Autodesk Inventor part; units mm, degrees
ref_plane "YZ Plane" through (0, 0, 0) normal (1, 0, 0) x (0, 1, 0)
ref_plane "XZ Plane" through (0, 0, 0) normal (0, 1, 0) x (-1, 0, 0)
ref_plane "XY Plane" through (0, 0, 0) normal (0, 0, 1) x (1, 0, 0)
sketch "Boceto1" plane through (0, 0, 0) normal (0, 0, 1) x (1, 0, 0)
  line L0 (48.5, -35) -> (48.5, 68)
  line L1 (48.5, 65) -> (35.5, 65)
  line L2 (-48.5, 68) -> (-48.5, -35)
  line L3 (-48.5, -32) -> (48.5, -32)
  line L4 (-48.5, -32) -> (48.5, -32)
  line L5 (48.5, -32) -> (48.5, 65)
  line L6 (48.5, 65) -> (-48.5, 65)
  line L7 (-48.5, 65) -> (-48.5, -32)
  point P0 (0, 0)
  point P1 (-48.5, 65)
extrude "Extrusión1" add sketch "Boceto1" along normal blind 3
sketch "Boceto5" plane through (0, 0, 0) normal (0, 0, -1) x (-1, 0, 0)
  line L0 (11.3801, -12.7901) -> (-11.3717, -12.7901)
  line L1 (19.791, -21.201) -> (5.6217, -7.0317)
  line L2 (-5.6132, -7.0317) -> (-19.7826, -21.201)
  line L3 (9.0613, -10.4713) -> (-9.0529, -10.4713)
  arc A0 (-19.7826, -21.201) -> (19.791, -21.201) centre (0.0042, 0) ccw
  point P0 (0, 0)
extrude "Extrusión5" cut sketch "Boceto5" against normal through all
sketch "Boceto6" plane through (0, 0, 0) normal (0, 0, -1) x (-1, 0, 0)
  arc A0 (-19.7826, -21.201) -> (19.791, -21.201) centre (0.0042, 0) ccw
  circle A1 centre (-38.9983, 5) radius 1.25
  circle A2 centre (-38.9983, 5) radius 1.25
  circle A3 centre (-38.9983, -5) radius 1.25
  circle A4 centre (39.0017, 5) radius 1.25
  circle A5 centre (39.0017, 5) radius 1.25
  circle A6 centre (39.0017, -5) radius 1.25
  point P0 (0, 0)
hole "Agujero1" at (-0.0042, 0, 0) direction (0, 0, 1) diameter 8.1 end through all
sketch "Boceto7" plane through (0, 0, 0) normal (0, 0, -1) x (-1, 0, 0)
  circle A0 centre (25.3722, 27.0019) radius 1.5
  circle A1 centre (0.0042, 0) radius 4.05
  arc A2 (-19.7826, -21.201) -> (19.791, -21.201) centre (0.0042, 0) ccw
  line L0 (-19.7826, -21.201) -> (-9.0529, -10.4713)
  line L1 (-9.0529, -10.4713) -> (9.0613, -10.4713)
  line L2 (9.0613, -10.4713) -> (19.791, -21.201)
  line L3 (48.5, 65) -> (48.5, -32)
  line L4 (-48.5, 65) -> (48.5, 65)
  line L5 (-48.5, -32) -> (-48.5, 65)
  line L6 (48.5, -32) -> (-48.5, -32)
  circle A3 centre (-25.3678, 26.9981) radius 1.5
  circle A4 centre (-25.3638, -27.0019) radius 1.25
  circle A5 centre (25.3762, -26.9981) radius 1.25
  circle A6 centre (-42, 58.5) radius 1.25
  circle A7 centre (42, 58.5) radius 1.25
  circle A8 centre (-38.9983, 5) radius 1.25
  circle A9 centre (-38.9983, 5) radius 1.25
  circle A10 centre (-38.9983, -5) radius 1.25
  circle A11 centre (39.0017, -5) radius 1.25
  circle A12 centre (39.0017, 5) radius 1.25
  point P0 (0, 0)
hole "Agujero2" at (-25.3762, -26.9981, 0) at (25.3638, -27.0019, 0) at (25.3678, 26.9981, 0) at (-25.3722, 27.0019, 0) at (42, 58.5, 0) at (-42, 58.5, 0) at (38.9983, -5, 0) at (38.9983, 5, 0) at (-39.0017, -5, 0) at (-39.0017, 5, 0) direction (0, 0, 1) diameter 2.5 end through all
sketch "Boceto9" plane through (0, 0, 0) normal (0, 0, -1) x (-1, 0, 0)
  line L0 (48.5, 65) -> (48.5, 49)
  line L1 (48.5, 65) -> (48.5, -32)
  line L2 (48.5, 49) -> (45.5, 49)
  line L3 (45.5, 49) -> (45.5, 29)
  line L4 (45.5, 29) -> (48.5, 29)
  point P0 (0, 0)
  dimension "d32" = 16
  dimension "d33" = 3
  dimension "d34" = 20
extrude "Extrusión7" cut sketch "Boceto9" against normal blind 10
properties part number "Madera intermedia"
CAD build for the part. Positions are in the model's coordinates, mm. A direction names the side the tool comes from. Give positions to 0.01 mm unless a question says otherwise; leave off trailing zeros. Order: outer loops, then holes, each group sorted by start corner. A loop starts at its lowest first (then second) coordinate and runs counter-clockwise, first axis right, second up.
(1) Saw through at C-C, the plane y = 58.5. Give the cut face in (x, z).
(2) Saw through at B-B, the plane x = -42. Give the cut face in (y, z), then the cut area to 4 significant figures.
(3) Saw through at A-A, the plane y = 0. Give the cut face in (x, z).
(4) Flat gauge pin, fed straight in: pin 1 (1.5 mm diameter, centred on y = 35.5, z = 2, fed in from -X). Where does the tip first touch, or does it go through?
(5) Tool access for faces 4 (the cylindrical face through (0, -29, 1)), 5 (the flat face through (-47, 29, 1)), 6 (the flat face through (1, 65, 1)): list every direction of +Z, -Z, +X, -X, +Y, -Y with a clear straight run to the whole face (end or side of a thin tool).
(6) Drill centre lines: L1, parallel to X at y = 5, z = 0.9; L2, parallel to Y at x = -42, z = 1.1; L3, parallel to X at y = 0, z = 0.8. Where is each one in solid material? Low to high.
(7) Mould opens along X. For faces 1 (the flat face through (0, -10.471, 1)), 2 (the flat face through (-1, 17, 3)), 3 (the flat face through (-45.5, 39, 1)) say: released by +X, released by -X, zero draft, split by the parting line, or undercut.
(8) Saw through at D-D, the plane z = 0.6. State how many separate pieces and enclosed holes the cut face has, then the cut area to 3 significant figures.
Results found:
1. outline: (-48.5, 0) - (-43.25, 0) - (-43.25, 3) - (-48.5, 3) - close; (-40.75, 0) - (40.75, 0) - (40.75, 3) - (-40.75, 3) - close; (43.25, 0) - (48.5, 0) - (48.5, 3) - (43.25, 3) - close
2. outline: (-32, 0) - (57.25, 0) - (57.25, 3) - (-32, 3) - close; (59.75, 0) - (65, 0) - (65, 3) - (59.75, 3) - close
2. area: 283.5 mm2
3. outline: (-48.5, 0) - (-4.05, 0) - (-4.05, 3) - (-48.5, 3) - close; (4.05, 0) - (48.5, 0) - (48.5, 3) - (4.05, 3) - close
4. pin 1: stops at x = -45.5
5. face 4: +Z, -Z
5. face 5: +Z, -Z, -X
5. face 6: +Z, -Z, +X, -X, +Y
6. L1: x = -48.5 to -40.25, -37.75 to 37.75, 40.25 to 48.5
6. L2: y = -32 to 57.25, 59.75 to 65
6. L3: x = -48.5 to -4.05, 4.05 to 48.5
7. face 1: undercut
7. face 2: zero draft
7. face 3: released by -X
8. separate pieces: 1
8. enclosed holes: 12
8. area: 8,730 mm2
